The model under review builds one solid part; all positions refer to its coordinate system, in mm. Face numbers are marked on the shaded views. A direction names the side the tool comes from. Coordinates: 2 decimals unless noted, no trailing zeros. Loops run counter-clockwise (first coordinate to the right, second up) from the corner with the lowest first, then second, coordinate; pieces in that order, holes last. Notation, with made-up numbers: M -29,38.25 L -21,38.25 A18 cw -21,71.25 Z; hole C 6.5,-15 d4. An arc over 180 degrees is marked long. Use CSV: the item, a comma, the result in double quotes. Start each with the question number.
1. Add section B-B, the plane z = -30.5. State how many separate pieces and enclosed holes the cut face has, then the cut area to 3 significant figures.
2. Add section A-A, the plane x = 9. Write out the cut boundary in (y, z).
3. Add section C-C, the plane z = -20. Write out the cut boundary in (x, y), then the cut area to 3 significant figures.
4. For L1, parallel to X at y = 4.4, z = -6; L2, parallel to X at y = 3.9, z = -30.5; L3, parallel to X at y = 6.25, z = -3, list the stretches that pass through material, from the lowest coordinate up.
5. Tool access review of the marked faces 1 and 2: name each direction out of +Z, -Z, +X, -X, +Y, -Y from which nothing blocks a thin tool from reaching the whole face with its end or side.
6. Draft analysis for pull direction Z (two halves, no side actions). For the marked faces 3, 4 and 5, state which applies: +Z half, -Z half, draft (parallel to the pull), parting line (faces both ways), or undercut.
7. Clearance check with flat-ended pins moving along their axes: P1, Ø1.8, axis at x = 19, z = -4.5, coming from the +Y side; P2, Ø3.5, axis at x = 18, z = -6, coming from the -Y side; P3, Ø4, axis at y = 4.5, z = -19.5, coming from the +X side. State where each tip first meets the part, or that it passes through.
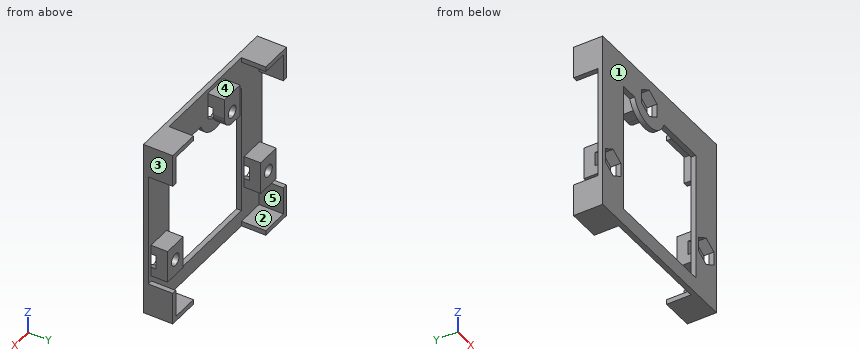
from build123d import *

# Parameters (mm, degrees)
SKETCH1_W           = 44
SKETCH1_H           = 44
SKETCH1_R           = 1.5
BOSS_EXTRUDE1_DEPTH = 1.2
BOSS_EXTRUDE4_DEPTH = 6
SKETCH5_W           = 6
SKETCH5_H           = 8
BOSS_EXTRUDE8_DEPTH = 4.1
SKETCH1_3_R         = 1.5
CUT_EXTRUDE1_DEPTH  = 2.5
SKETCH1_4_R         = 1.5
CUT_EXTRUDE2_DEPTH  = 63.640561939


with BuildPart() as part:
    # Sketch1 → Boss-Extrude1 (new body)
    # profile 1 of 4: a face of its own
    with BuildSketch(Plane(origin=(0, 0, 0), x_dir=(1, 0, 0), z_dir=(0, 1, 0))):
        with Locations((22, 22)):
            Rectangle(SKETCH1_W, SKETCH1_H)
        Polygon((18, 9.464101615), (15, 7.732050808), (15, 4.267949192), (18, 2.535898385), (21, 4.267949192), (21, 7.732050808), align=None, mode=Mode.SUBTRACT)
        Polygon((40, 33.964101615), (37, 32.232050808), (37, 28.767949192), (40, 27.035898385), (43, 28.767949192), (43, 32.232050808), align=None, mode=Mode.SUBTRACT)
        Polygon((4, 33.964101615), (1, 32.232050808), (1, 28.767949192), (4, 27.035898385), (7, 28.767949192), (7, 32.232050808), align=None, mode=Mode.SUBTRACT)
        with BuildLine():
            Line((23.656854249, 8), (36, 8))
            Line((36, 8), (36, 40))
            Line((36, 40), (8, 40))
            Line((8, 40), (8, 8))
            Line((8, 8), (12.343145751, 8))
            ThreePointArc((12.343145751, 8), (18, 12), (23.656854249, 8))
        make_face(mode=Mode.SUBTRACT)
    # profile 2 of 4: a face of its own
    with BuildSketch(Plane(origin=(0, 0, 0), x_dir=(1, 0, 0), z_dir=(0, 1, 0))):
        Polygon((21, 7.732050808), (18, 9.464101615), (15, 7.732050808), (15, 4.267949192), (18, 2.535898385), (21, 4.267949192), align=None)
        with Locations(Location((18, 6, 0), (0, 0, 270))):
            Circle(SKETCH1_R, mode=Mode.SUBTRACT)
    # profile 3 of 4: a face of its own
    with BuildSketch(Plane(origin=(0, 0, 0), x_dir=(1, 0, 0), z_dir=(0, 1, 0))):
        Polygon((43, 32.232050808), (40, 33.964101615), (37, 32.232050808), (37, 28.767949192), (40, 27.035898385), (43, 28.767949192), align=None)
        with Locations(Location((40, 30.5, 0), (0, 0, 270))):
            Circle(SKETCH1_R, mode=Mode.SUBTRACT)
    # profile 4 of 4: a face of its own
    with BuildSketch(Plane(origin=(0, 0, 0), x_dir=(1, 0, 0), z_dir=(0, 1, 0))):
        Polygon((7, 32.232050808), (4, 33.964101615), (1, 32.232050808), (1, 28.767949192), (4, 27.035898385), (7, 28.767949192), align=None)
        with Locations(Location((4, 30.5, 0), (0, 0, 270))):
            Circle(SKETCH1_R, mode=Mode.SUBTRACT)
    extrude(amount=BOSS_EXTRUDE1_DEPTH)

    # Sketch4 → Boss-Extrude4 (add)
    with BuildSketch(Plane(origin=(0, 1.2, 0), x_dir=(1, 0, 0), z_dir=(0, 1, 0))):
        Polygon((8, 44), (0, 44), (0, 36), (1.2, 36), (1.2, 42.8), (8, 42.8), align=None)
        Polygon((44, 44), (36, 44), (36, 42.8), (42.8, 42.8), (42.8, 36), (44, 36), align=None)
        Polygon((36, 0), (44, 0), (44, 8), (42.8, 8), (42.8, 1.2), (36, 1.2), align=None)
        Polygon((0, 0), (8, 0), (8, 1.2), (1.2, 1.2), (1.2, 8), (0, 8), align=None)
    extrude(amount=BOSS_EXTRUDE4_DEPTH)

    # Sketch5 → Boss-Extrude8 (add)
    with BuildSketch(Plane(origin=(0, 1.2, 0), x_dir=(1, 0, 0), z_dir=(0, 1, 0))):
        with Locations((4, 30.5)):
            Rectangle(SKETCH5_W, SKETCH5_H)
        with Locations((40, 30.5)):
            Rectangle(SKETCH5_W, SKETCH5_H)
        with BuildLine():
            Line((15, 9), (18, 9))
            ThreePointArc((18, 9), (20.121320344, 8.121320344), (21, 6))
            Line((21, 6), (21, 1))
            Line((21, 1), (15, 1))
            Line((15, 1), (15, 9))
        make_face()
    extrude(amount=BOSS_EXTRUDE8_DEPTH)

    # Sketch1_3 → Cut-Extrude1 (cut)
    # profile 1 of 3: a face of its own
    with BuildSketch(Plane(origin=(0, 0, 0), x_dir=(1, 0, 0), z_dir=(0, 1, 0))):
        Polygon((7, 32.232050808), (4, 33.964101615), (1, 32.232050808), (1, 28.767949192), (4, 27.035898385), (7, 28.767949192), align=None)
        with Locations(Location((4, 30.5, 0), (0, 0, 270))):
            Circle(SKETCH1_3_R, mode=Mode.SUBTRACT)
    # profile 2 of 3: a face of its own
    with BuildSketch(Plane(origin=(0, 0, 0), x_dir=(1, 0, 0), z_dir=(0, 1, 0))):
        Polygon((21, 7.732050808), (18, 9.464101615), (15, 7.732050808), (15, 4.267949192), (18, 2.535898385), (21, 4.267949192), align=None)
        with Locations(Location((18, 6, 0), (0, 0, 90))):
            Circle(SKETCH1_3_R, mode=Mode.SUBTRACT)
    # profile 3 of 3: a face of its own
    with BuildSketch(Plane(origin=(0, 0, 0), x_dir=(1, 0, 0), z_dir=(0, 1, 0))):
        Polygon((43, 32.232050808), (40, 33.964101615), (37, 32.232050808), (37, 28.767949192), (40, 27.035898385), (43, 28.767949192), align=None)
        with Locations(Location((40, 30.5, 0), (0, 0, 270))):
            Circle(SKETCH1_3_R, mode=Mode.SUBTRACT)
    extrude(amount=CUT_EXTRUDE1_DEPTH, mode=Mode.SUBTRACT)

    # Sketch1_4 → Cut-Extrude2 (cut, through all)
    with BuildSketch(Plane(origin=(0, 0, 0), x_dir=(1, 0, 0), z_dir=(0, 1, 0))):
        with Locations(Location((4, 30.5, 0), (0, 0, 270))):
            Circle(SKETCH1_4_R)
        with Locations(Location((18, 6, 0), (0, 0, 90))):
            Circle(SKETCH1_4_R)
        with Locations(Location((40, 30.5, 0), (0, 0, 270))):
            Circle(SKETCH1_4_R)
    extrude(amount=CUT_EXTRUDE2_DEPTH, mode=Mode.SUBTRACT)


solid = part.part
Computed:
1,separate pieces,"8"
1,enclosed holes,"0"
1,area,"21.6 mm^2"
2,outline,"M 0,-44 L 1.2,-44 L 1.2,-40 L 0,-40 Z; M 0,-8 L 1.2,-8 L 1.2,0 L 0,0 Z"
3,outline,"M 0,0 L 8,0 L 8,1.2 L 0,1.2 Z; M 36,0 L 44,0 L 44,1.2 L 36,1.2 Z"
3,area,"19.2 mm^2"
4,L1,"x = 0 to 1.2, 15 to 16.5, 19.5 to 21, 42.8 to 44"
4,L2,"x = 1 to 2.5, 5.5 to 7, 37 to 38.5, 41.5 to 43"
4,L3,"x = 0 to 1.2, 42.8 to 44"
5,face 1,"+Z, -Z, +X, -X, -Y"
5,face 2,"+Y"
6,face 3,"draft"
6,face 4,"+Z half"
6,face 5,"undercut"
7,P1,"stops at y = 5.3"
7,P2,"stops at y = 2.5"
7,P3,"passes through"
